Could you check a few things on this model? Use its own coordinates, in mm. Coordinates: 2 decimals unless noted, no trailing zeros. Loops run counter-clockwise (first coordinate to the right, second up) from the corner with the lowest first, then second, coordinate; pieces in that order, holes last. Notation, with made-up numbers: (7.25, 11.25) - (51.25, 11.25) arc R13 ccw to (51.25, 22.25) - close; hole circle Ø2 at (59, -1). An arc over 180 degrees is marked (long way). One line per item, written item: value. Start each with the question number.
(1) If we mould it in two halves opening along X, with no side actions, what happens to faces 1 (the face through (-11.94, 2.96, 26.99)), 2 (the face through (14, 6, -8)), 3 (the face through (81.724, 3.042, -6.268))? For each: pulls with the +X half, pulls with the -X half, needs draft (parallel to the pull), parting line crosses it, or undercut.
(2) If I drill on line 1 along Z through (x, y) = (25, 4.5); line 2 along Z through (x, y) = (75.5, 1.4); line 3 along X through (y, z) = (5, -29), over which ranges is the centre line in solid material (lowest first)? Write a range as from..to.
(3) If we section it at A-A on y = 2.55: Write out the boundary of the cut face in (x, z), then the cut area to 3 significant figures.
(4) If we section it at C-C on z = -23: Write out the boundary of the cut face in (x, y).
(5) If we section it at B-B on x = 56: Write out the boundary of the cut face in (y, z), then the cut area to 3 significant figures.
(6) I'm going to push flat-ended pins straight in: P1, Ø1.5, axis at y = 1.5, z = -1.5, coming from the +X side; P2, Ø1, axis at x = 13.5, y = 4, coming from the +Z side; P3, Ø3, axis at y = 1, z = -34, coming from the +X side. Where does each tip first touch, or does it pass through?
```python
from build123d import *

# Parameters (mm, degrees)
SKETCH1_R           = 4.5
SKETCH1_R_2         = 44.53
BOSS_EXTRUDE1_DEPTH = 6
SKETCH2_R           = 1.5
CUT_EXTRUDE1_DEPTH  = 10


with BuildPart() as part:
    # Sketch1 → Boss-Extrude1 (new body)
    # profile 1 of 7: a face of its own
    with BuildSketch(Plane(origin=(0, 0, 0), x_dir=(1, 0, 0), z_dir=(0, 1, 0))):
        with BuildLine():
            Line((3.706249193, 49.435224426), (-27.146075319, 33.07485149))
            ThreePointArc((-27.146075319, 33.07485149), (-53.146075319, 7.07485149), (-27.146075319, -18.92514851))
            Line((-27.146075319, -18.92514851), (3.706249193, -35.285521446))
            ThreePointArc((3.706249193, -35.285521446), (-4.027102695, -28.958383674), (-10.375107984, -21.242151909))
            Line((-10.375107984, -21.242151909), (-27.146075319, -13.92514851))
            ThreePointArc((-27.146075319, -13.92514851), (-48.146075319, 7.07485149), (-27.146075319, 28.07485149))
            Line((-27.146075319, 28.07485149), (-9.910194417, 36.074047649))
            ThreePointArc((-9.910194417, 36.074047649), (-3.73365085, 43.398382562), (3.706249193, 49.435224426))
        make_face()
    # profile 2 of 7: a face of its own
    with BuildSketch(Plane(origin=(0, 0, 0), x_dir=(1, 0, 0), z_dir=(0, 1, 0))):
        with BuildLine():
            ThreePointArc((-10.375107984, -21.242151909), (-18.97940126, 7.487626122), (-9.910194417, 36.074047649))
            Line((-9.910194417, 36.074047649), (-27.146075319, 28.07485149))
            ThreePointArc((-27.146075319, 28.07485149), (-48.146075319, 7.07485149), (-27.146075319, -13.92514851))
            Line((-27.146075319, -13.92514851), (-10.375107984, -21.242151909))
        make_face()
        with Locations(Location((-27.146075319, 7.07485149, 0), (0, 0, 270))):
            Circle(SKETCH1_R, mode=Mode.SUBTRACT)
    # profile 3 of 7: a face of its own
    with BuildSketch(Plane(origin=(0, 0, 0), x_dir=(1, 0, 0), z_dir=(0, 1, 0))):
        with BuildLine():
            ThreePointArc((82.798924681, 7.07485149), (55.935555161, 51.935893919), (3.706249193, 49.435224426))
            ThreePointArc((3.706249193, 49.435224426), (-3.73365085, 43.398382562), (-9.910194417, 36.074047649))
            Line((-9.910194417, 36.074047649), (6.70287652, 43.784196842))
            ThreePointArc((6.70287652, 43.784196842), (52.651339866, 46.478824796), (76.438924681, 7.07485149))
            ThreePointArc((76.438924681, 7.07485149), (50.975331795, -33.166831126), (3.706249193, -27.385705604))
            Line((3.706249193, -27.385705604), (-10.375107984, -21.242151909))
            ThreePointArc((-10.375107984, -21.242151909), (-4.027102695, -28.958383674), (3.706249193, -35.285521446))
            ThreePointArc((3.706249193, -35.285521446), (55.935555161, -37.786190939), (82.798924681, 7.07485149))
        make_face()
    # profile 4 of 7: a face of its own
    with BuildSketch(Plane(origin=(0, 0, 0), x_dir=(1, 0, 0), z_dir=(0, 1, 0))):
        with BuildLine():
            Line((6.70287652, 43.784196842), (-9.910194417, 36.074047649))
            ThreePointArc((-9.910194417, 36.074047649), (-18.97940126, 7.487626122), (-10.375107984, -21.242151909))
            Line((-10.375107984, -21.242151909), (3.706249193, -27.385705604))
            ThreePointArc((3.706249193, -27.385705604), (-12.581655153, 8.948138973), (6.70287652, 43.784196842))
        make_face()
    # profile 5 of 7: a face of its own
    with BuildSketch(Plane(origin=(0, 0, 0), x_dir=(1, 0, 0), z_dir=(0, 1, 0))):
        with BuildLine():
            ThreePointArc((82.798924681, 7.07485149), (55.935555161, 51.935893919), (3.706249193, 49.435224426))
            ThreePointArc((3.706249193, 49.435224426), (-3.73365085, 43.398382562), (-9.910194417, 36.074047649))
            Line((-9.910194417, 36.074047649), (6.70287652, 43.784196842))
            ThreePointArc((6.70287652, 43.784196842), (52.651339866, 46.478824796), (76.438924681, 7.07485149))
            ThreePointArc((76.438924681, 7.07485149), (50.975331795, -33.166831126), (3.706249193, -27.385705604))
            Line((3.706249193, -27.385705604), (-10.375107984, -21.242151909))
            ThreePointArc((-10.375107984, -21.242151909), (-4.027102695, -28.958383674), (3.706249193, -35.285521446))
            ThreePointArc((3.706249193, -35.285521446), (55.935555161, -37.786190939), (82.798924681, 7.07485149))
        make_face()
    # profile 6 of 7: a face of its own
    with BuildSketch(Plane(origin=(0, 0, 0), x_dir=(1, 0, 0), z_dir=(0, 1, 0))):
        with BuildLine():
            Line((6.70287652, 43.784196842), (-9.910194417, 36.074047649))
            ThreePointArc((-9.910194417, 36.074047649), (-18.97940126, 7.487626122), (-10.375107984, -21.242151909))
            Line((-10.375107984, -21.242151909), (3.706249193, -27.385705604))
            ThreePointArc((3.706249193, -27.385705604), (-12.581655153, 8.948138973), (6.70287652, 43.784196842))
        make_face()
    # profile 7 of 7: a face of its own
    with BuildSketch(Plane(origin=(0, 0, 0), x_dir=(1, 0, 0), z_dir=(0, 1, 0))):
        with Locations((31.908924681, 7.07485149)):
            Circle(SKETCH1_R_2)
        with Locations(Location((31.908924681, 7.07485149, 0), (0, 0, 270))):
            Circle(SKETCH1_R, mode=Mode.SUBTRACT)
    extrude(amount=BOSS_EXTRUDE1_DEPTH)

    # Sketch2 → Cut-Extrude1 (cut)
    with BuildSketch(Plane(origin=(0, 6, 0), x_dir=(1, 0, 0), z_dir=(0, 1, 0))):
        with Locations(Location((-50.446075319, 7.07485149, 0), (0, 0, 270))):
            Circle(SKETCH2_R)
        with Locations(Location((80.458924681, 7.07485149, 0), (0, 0, 270))):
            Circle(SKETCH2_R)
    extrude(amount=-CUT_EXTRUDE1_DEPTH, mode=Mode.SUBTRACT)


solid = part.part
```
Values:
1. face 1: pulls with the -X half
1. face 2: needs draft
1. face 3: undercut
2. line 1: z = -57.49..43.34
2. line 2: z = -33.34..19.19
2. line 3: x = -41.12..77.83
3. outline: (-27.15, -33.07) - (3.71, -49.44) arc R50.89 ccw (long way) to (3.71, 35.29) - (-27.15, 18.93) arc R26 ccw to start; hole circle Ø3 at (-50.45, -7.07); hole circle Ø9 at (-27.15, -7.07); hole circle Ø9 at (31.91, -7.07); hole circle Ø3 at (80.46, -7.07)
3. area: 9,810 mm2
4. outline: (-47.7, 0) - (80.24, 0) - (80.24, 6) - (-47.7, 6) - close
5. outline: (0, -51.9) - (6, -51.9) - (6, 37.75) - (0, 37.75) - close
5. area: 538 mm2
6. P1: stops at x = 82.57
6. P2: stops at z = 40.56
6. P3: stops at x = 75.99
